Answer from the drawing. Dimensions are ordinates in mm from the lowest x, y and z of the part. Coordinates: 2 decimals unless noted, no trailing zeros. Order: outer loops, then holes, each group sorted by start corner. A loop starts at its lowest first (then second) coordinate and runs counter-clockwise, first axis right, second up. Notation, with made-up numbers: (-2, 4.5) -> (34, 4.5) arc R29 ccw to (34, 36.5) -> close; hole circle Ø2 at (-9, 20.25). An arc over 180 degrees is marked (long way). Use CSV: the item, a comma, the result in double quotes.
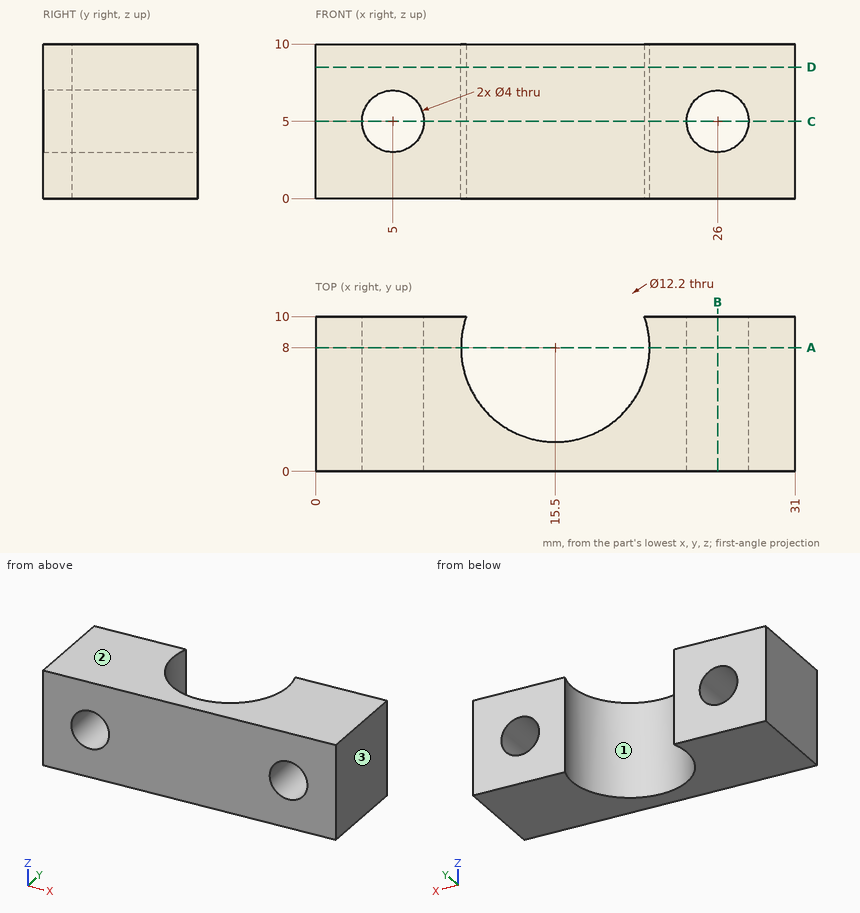
Item 1: The mould has two halves that part along X. Classify the marked faces 1, 2 and 3: +X half, -X half, draft (parallel to the pull), parting line (faces both ways), or undercut.
Return value:
face 1,"undercut"
face 2,"draft"
face 3,"+X half"
Item 2: Find section C-C, the plane z = 5. Give the vertices of the cut face in (x, y), then the cut area to 3 significant figures.
Return value:
outline,"(0, 0) -> (3, 0) -> (3, 10) -> (0, 10) -> close; (7, 0) -> (24, 0) -> (24, 10) -> (21.26, 10) arc R6.1 cw (long way) to (9.74, 10) -> (7, 10) -> close; (28, 0) -> (31, 0) -> (31, 10) -> (28, 10) -> close"
area,"148 mm^2"
Item 3: Find section A-A, the plane y = 8. Give the vertices of the cut face in (x, z), then the cut area to 3 significant figures.
Return value:
outline,"(0, 0) -> (9.4, 0) -> (9.4, 10) -> (0, 10) -> close; (21.6, 0) -> (31, 0) -> (31, 10) -> (21.6, 10) -> close; hole circle Ø4 at (5, 5); hole circle Ø4 at (26, 5)"
area,"163 mm^2"
Item 4: Find section B-B, the plane x = 26. Give the vertices of the cut face in (y, z).
Return value:
outline,"(0, 0) -> (10, 0) -> (10, 3) -> (0, 3) -> close; (0, 7) -> (10, 7) -> (10, 10) -> (0, 10) -> close"
Item 5: Find section D-D, the plane z = 8.5. Give the vertices of the cut face in (x, y).
Return value:
outline,"(0, 0) -> (31, 0) -> (31, 10) -> (21.26, 10) arc R6.1 cw (long way) to (9.74, 10) -> (0, 10) -> close"
Item 6: Straight lines are drawn through the part: line 1 along X through (y, z) = (6.5, 4.25); line 2 along X through (y, z) = (3.25, 5); line 3 along X through (y, z) = (8, 7.5). For each, find the intervals that lie inside material, in ascending order.
Return value:
line 1,"x = 0 to 3.15, 6.85 to 9.59, 21.41 to 24.15, 27.85 to 31"
line 2,"x = 0 to 3, 7 to 11.67, 19.33 to 24, 28 to 31"
line 3,"x = 0 to 9.4, 21.6 to 31"
